The listing builds one solid part. Answer for the finished solid, in the listing's coordinates (mm). Face numbers are marked on the shaded views. A direction names the side the tool comes from. Give positions to 0.01 mm unless a question says otherwise; leave off trailing zeros. Order: outer loops, then holes, each group sorted by start corner. A loop starts at its lowest first (then second) coordinate and runs counter-clockwise, first axis right, second up. Notation, with made-up numbers: (89, 59.5) - (97, 59.5) arc R11 cw to (97, 64.5) - close; hole circle Ø2 at (-15, 58.25). An arc over 180 degrees is marked (long way). Write each question's results on one line, items separated by ' | '. Start each with the question number.
1. Which of the six approach directions +Z, -Z, +X, -X, +Y, -Y give full straight-line access (tool end or side, diameter ignored) to the marked faces 5 and 6?
2. Section B-B (x = 5) is taken. Give the vertices of the cut face in (y, z), and give its area (3 significant figures).
3. Section C-C (z = 17.25) is taken. Give the vertices of the cut face in (x, y).
4. Section A-A (z = 21.75) is taken. Give the vertices of the cut face in (x, y).
5. Find the intervals of material crossed by L1, parallel to Y at x = 6.5, z = 20.5; L2, parallel to Y at x = 7, z = 21.75; L3, parallel to Y at x = 19.5, z = 30.5, in increasing order.
6. Determine the mould class of the marked faces 1, 2, 3 and 4 for opening direction Y: released by +Y, released by -Y, zero draft, split by the parting line, or undercut.
7. Section D-D (y = -8.5) is taken. Give the vertices of the cut face in (x, z).
8. Flat-ended cylindrical pins translate along their axes: pin 1 (7 mm diameter, centred on y = 20.95, z = 20.95, fed in from +X); pin 2 (3 mm diameter, centred on x = 21, z = 23.5, fed in from -Y); pin 3 (3 mm diameter, centred on x = 34, z = 22.5, fed in from +Y); pin 4 (2.5 mm diameter, centred on y = 20.95, z = 20.95, fed in from +X). Find the tip coordinate at first contact, or state that the pin passes through.
Autodesk Inventor part; units mm, degrees
ref_plane "YZ Plane" through (0, 0, 0) normal (1, 0, 0) x (0, 1, 0)
ref_plane "XZ Plane" through (0, 0, 0) normal (0, 1, 0) x (-1, 0, 0)
ref_plane "XY Plane" through (0, 0, 0) normal (0, 0, 1) x (1, 0, 0)
sketch "Sketch1" plane through (0, 0, 0) normal (1, 0, 0) x (0, 1, 0)
  arc A0 (31.1103, 13.7167) -> (-31.1103, 13.7167) centre (0, 0) ccw
  arc A1 (20.4522, 13.7167) -> (-20.4522, 13.7167) centre (0, 0) ccw
  line L0 (0, 0) -> (34, 0) construction
  circle A2 centre (20.9487, 20.9487) radius 1.5
  line L1 (31.1103, 13.7167) -> (20.4522, 13.7167)
  line L2 (-20.4522, 13.7167) -> (-31.1103, 13.7167)
  line L3 (0, 0) -> (34, 0) construction
  circle A3 centre (-20.9487, 20.9487) radius 1.5
extrude "Extrusion1" add sketch "Sketch1" along normal blind 8
sketch "Sketch2" plane through (8, 0, 0) normal (1, 0, 0) x (0, 0, -1)
  circle A0 centre (-20.9487, 20.9487) radius 1.5
  circle A1 centre (-20.9487, 20.9487) radius 3
  circle A2 centre (-20.9487, -20.9487) radius 1.5
  circle A3 centre (-20.9487, -20.9487) radius 3
  point P0 (0, 0)
  dimension "d8" = 6
extrude "Extrusion2" cut sketch "Sketch2" against normal blind 4
sketch "Sketch3" plane through (8, 0, 0) normal (1, 0, 0) x (0, 0, -1)
  line L0 (-20.1744, 14.1221) -> (-30.9284, 14.1221)
  arc A0 (-13.7167, 31.1103) -> (-13.7167, -31.1103) centre (0, 0) ccw
  line L1 (-20.1744, -14.1221) -> (-30.9284, -14.1221)
  arc A1 (-30.9284, 14.1221) -> (-30.9284, -14.1221) centre (0, 0) ccw
  line L2 (-20.1744, 14.1221) -> (-20.1744, -14.1221)
extrude "Extrusion3" add sketch "Sketch3" along normal blind 40
properties part number "Lid_Tilt"
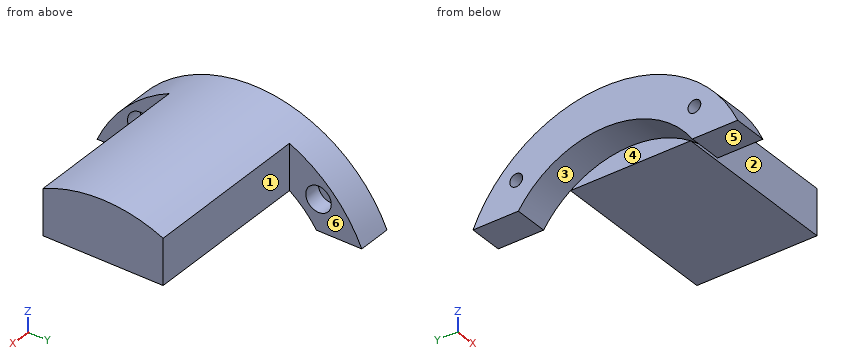
Reported:
1) face 5: -Z, +X, -X, +Y, -Y | face 6: +Z, -Z, +X, +Y
2) outline: (-31.11, 13.72) - (-20.45, 13.72) arc R24.63 cw to (20.45, 13.72) - (31.11, 13.72) arc R34 ccw to start; hole circle Ø6 at (-20.95, 20.95); hole circle Ø6 at (20.95, 20.95) | area: 539 mm²
3) outline: (0, -29.3) - (8, -29.3) - (8, -17.57) - (0, -17.57) - close; (0, 17.57) - (8, 17.57) - (8, 29.3) - (0, 29.3) - close
4) outline: (0, -26.13) - (8, -26.13) - (8, -23.84) - (4, -23.84) - (4, -22.22) - (0, -22.22) - close; (0, -19.68) - (4, -19.68) - (4, -18.06) - (8, -18.06) - (8, -14.12) - (48, -14.12) - (48, 14.12) - (8, 14.12) - (8, 18.06) - (4, 18.06) - (4, 19.68) - (0, 19.68) - (0, 11.55) - (8, 11.55) - (8, -11.55) - (0, -11.55) - close; (0, 22.22) - (4, 22.22) - (4, 23.84) - (8, 23.84) - (8, 26.13) - (0, 26.13) - close
5) L1: -27.12 to -23.91, -17.98 to -13.65, 13.65 to 17.98, 23.91 to 27.12 | L2: -26.13 to -23.84, -18.06 to -11.55, 11.55 to 18.06, 23.84 to 26.13 | L3: -14.12 to 14.12
6) face 1: released by +Y | face 2: released by -Y | face 3: undercut | face 4: undercut
7) outline: (0, 23.11) - (8, 23.11) - (8, 20.17) - (48, 20.17) - (48, 32.92) - (0, 32.92) - close
8) pin 1: x = 8 | pin 2: y = -14.12 | pin 3: y = 14.12 | pin 4: through
